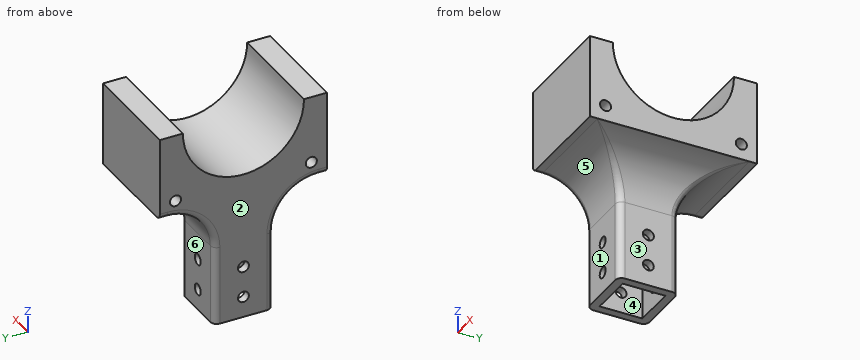
```python
from build123d import *

# Parameters (mm, degrees)
SKETCH_1_W          = 28.5
SKETCH_1_H          = 28.5
SKETCH_1_W_2        = 20.5
SKETCH_1_H_2        = 20.5
EXTRUDE_1_DEPTH     = 30
SKETCH_2_W          = 80
SKETCH_2_H          = 80
SKETCH_2_R          = 29
EXTRUDE_2_DEPTH     = 51
FILLET_1_R          = 22
CUT_EXTRUDE_1_DEPTH = 51
SKETCH_5_W          = 28.5
SKETCH_5_H          = 28.5
SKETCH_5_W_2        = 20.5
SKETCH_5_H_2        = 20.5
EXTRUDE_3_DEPTH     = 30
SKETCH_6_R          = 2.6
SKETCH_6_R_2        = 2.65
CUT_EXTRUDE_2_DEPTH = 30
SKETCH_7_R          = 2.65
CUT_EXTRUDE_3_DEPTH = 30
SKETCH_8_R          = 2.65
CUT_EXTRUDE_4_DEPTH = 96.399161422
FILLET_3_R          = 3


with BuildPart() as part:
    # 草图1 → 凸台-拉伸1 (new body)
    with BuildSketch(Plane.XY):
        Rectangle(SKETCH_1_W, SKETCH_1_H)
        Rectangle(SKETCH_1_W_2, SKETCH_1_H_2, mode=Mode.SUBTRACT)
    extrude(amount=EXTRUDE_1_DEPTH)

    # 草图2 → 凸台-拉伸2 (add)
    with BuildSketch(Plane.ZY.offset(14.25)):
        with Locations((70, 0)):
            Rectangle(SKETCH_2_W, SKETCH_2_H)
        with Locations((70, 0)):
            Circle(SKETCH_2_R, mode=Mode.SUBTRACT)
    extrude(amount=-EXTRUDE_2_DEPTH)

    # 圆角1
    fillet_1_edges = [part.edges().sort_by_distance(p)[0] for p in [
        (14.25, 0, 30),
        (0, 14.25, 30),
        (0, -14.25, 30),
    ]]
    fillet(fillet_1_edges, radius=FILLET_1_R)

    # 草图3 → 切除-拉伸1 (cut)
    with BuildSketch(Plane.ZY.offset(14.25)):
        with BuildLine():
            Line((70, -29), (70, -40))
            Line((70, -40), (110, -40))
            Line((110, -40), (110, 40))
            Line((110, 40), (70, 40))
            Line((70, 40), (70, 29))
            ThreePointArc((70, 29), (90.506096654, 20.506096654), (99, 0))
            ThreePointArc((99, 0), (90.506096654, -20.506096654), (70, -29))
        make_face()
    extrude(amount=-CUT_EXTRUDE_1_DEPTH, mode=Mode.SUBTRACT)

    # 草图5 → 凸台-拉伸3 (add)
    with BuildSketch(Plane(origin=(0, 0, 0), x_dir=(-1, 0, 0), z_dir=(0, 0, -1))):
        Rectangle(SKETCH_5_W, SKETCH_5_H)
        Rectangle(SKETCH_5_W_2, SKETCH_5_H_2, mode=Mode.SUBTRACT)
    extrude(amount=EXTRUDE_3_DEPTH)

    # 草图6 → 切除-拉伸2 (cut)
    with BuildSketch(Plane(origin=(14.25, 0, 0), x_dir=(0, 0, -1), z_dir=(1, 0, 0))):
        with Locations((20, 0)):
            Circle(SKETCH_6_R)
        with Locations((5, 0)):
            Circle(SKETCH_6_R_2)
    extrude(amount=-CUT_EXTRUDE_2_DEPTH, mode=Mode.SUBTRACT)

    # 草图7 → 切除-拉伸3 (cut)
    with BuildSketch(Plane(origin=(0, 14.25, 0), x_dir=(1, 0, 0), z_dir=(0, 1, 0))):
        with Locations(Location((0, 20, 0), (0, 0, 270))):
            Circle(SKETCH_7_R)
        with Locations(Location((0, 5, 0), (0, 0, 270))):
            Circle(SKETCH_7_R)
    extrude(amount=-CUT_EXTRUDE_3_DEPTH, mode=Mode.SUBTRACT)

    # 草图8 → 切除-拉伸4 (cut, through all)
    with BuildSketch(Plane.ZY.offset(14.25)):
        with Locations((37.5, 32.5)):
            Circle(SKETCH_8_R)
        with Locations((37.5, -32.5)):
            Circle(SKETCH_8_R)
    extrude(amount=-CUT_EXTRUDE_4_DEPTH, mode=Mode.SUBTRACT)

    # 圆角3
    fillet_3_edges = [part.edges().sort_by_distance(p)[0] for p in [
        (-14.25, -38.125, 30),
        (-14.25, 38.125, 30),
        (14.25, -14.25, -11),
        (-14.25, -14.25, -11),
        (14.25, 14.25, -11),
        (-14.25, 14.25, -11),
        (-14.25, -20.693650814, 23.556349186),
        (-14.25, 20.693650814, 23.556349186),
        (22.036924037, 22.036924037, 24.792512369),
        (22.036924037, -22.036924037, 24.792512369),
    ]]
    fillet(fillet_3_edges, radius=FILLET_3_R)


solid = part.part
```
Design review of the part built by this model. Coordinates are the model's own, in mm. Face numbers are marked on the shaded views. A direction names the side the tool comes from. Coordinates: 2 decimals unless noted, no trailing zeros. Order: outer loops, then holes, each group sorted by start corner. A loop starts at its lowest first (then second) coordinate and runs counter-clockwise, first axis right, second up. Notation, with made-up numbers: M 72.5,17.5 L 84.5,17.5 A31 cw 84.5,55.5 Z; hole C 58,59 d7. An arc over 180 degrees is marked long. Answer as a JSON object with one key per item and string values. Group by question number.
1) For pin 1 (4 mm diameter, centred on x = 0, z = -5, fed in from -Y); pin 2 (7 mm diameter, centred on x = 0, z = -20, fed in from -Y); pin 3 (6 mm diameter, centred on x = 3, z = 8.5, fed in from -Y); pin 4 (6 mm diameter, centred on y = -0.5, z = 10.5, fed in from +X), all flat-tipped, find the tip position at first contact; note any pin that passes through.
2) Add section A-A, the plane x = 0. Count the separate pieces of the cut face and the enclosed holes in it, then the cut area to 3 significant figures.
3) Mouldability with a two-part tool opening along X and no side actions: class the marked faces 1, 2, 3 and 4 as pulls with the +X half, pulls with the -X half, needs draft (parallel to the pull), parting line crosses it, or undercut.
4) Add section C-C, the plane z = -5. Write out the cut boundary in (x, y), then the cut area to 3 significant figures.
5) Add section B-B, the plane y = 0. Write out the cut boundary in (x, z).
6) Wall thickness on L1, parallel to Y at x = -0.5, z = -13; L2, parallel to Z at x = 4, y = 34.5; L3, parallel to Y at x = 12, z = -5: over which ranges is each line inside the solid? List them lowest first.
7) Add section D-D, the plane x = -8. Write out the cut boundary in (y, z), then the cut area to 3 significant figures.
8) Tool access review of the marked faces 5 and 6: name each direction out of +Z, -Z, +X, -X, +Y, -Y from which nothing blocks a thin tool from reaching the whole face with its end or side.
Computed values:
{
 "1": {"pin 1": "passes through", "pin 2": "stops at y = -14.25", "pin 3": "stops at y = -14.53", "pin 4": "stops at x = 14.95"},
 "2": {"separate pieces": "5", "enclosed holes": "2", "area": "2,440 mm^2"},
 "3": {"face 1": "needs draft", "face 2": "pulls with the -X half", "face 3": "pulls with the +X half", "face 4": "undercut"},
 "4": {"outline": "M -14.25,-11.25 A3 ccw -11.25,-14.25 L -2.65,-14.25 L -2.65,-10.25 L -10.25,-10.25 L -10.25,-2.65 L -14.25,-2.65 Z; M -14.25,2.65 L -10.25,2.65 L -10.25,10.25 L -2.65,10.25 L -2.65,14.25 L -11.25,14.25 A3 ccw -14.25,11.25 Z; M 2.65,-14.25 L 11.25,-14.25 A3 ccw 14.25,-11.25 L 14.25,-2.65 L 10.25,-2.65 L 10.25,-10.25 L 2.65,-10.25 Z; M 2.65,10.25 L 10.25,10.25 L 10.25,2.65 L 14.25,2.65 L 14.25,11.25 A3 ccw 11.25,14.25 L 2.65,14.25 Z", "area": "299 mm^2"},
 "5": {"outline": "M -14.25,-30 L -10.25,-30 L -10.25,-22.6 L -14.25,-22.6 Z; M -14.25,-17.4 L -10.25,-17.4 L -10.25,-7.65 L -14.25,-7.65 Z; M -14.25,-2.35 L -10.25,-2.35 L -10.25,30 L 10.25,30 L 10.25,-2.35 L 14.25,-2.35 L 14.25,8 A22 cw 36.25,30 L 36.75,30 L 36.75,41 L -14.25,41 Z; M 10.25,-30 L 14.25,-30 L 14.25,-22.6 L 10.25,-22.6 Z; M 10.25,-17.4 L 14.25,-17.4 L 14.25,-7.65 L 10.25,-7.65 Z"},
 "6": {"L1": "y = -14.25 to -10.25, 10.25 to 14.25", "L2": "z = 29.93 to 35.76, 39.24 to 70", "L3": "y = -14.15 to -2.65, 2.65 to 14.15"},
 "7": {"outline": "M -40,30 L -36.25,30 A22 cw -14.25,8 L -14.25,-30 L -10.25,-30 L -10.25,30 L 10.25,30 L 10.25,-30 L 14.25,-30 L 14.25,8 A22 cw 36.25,30 L 40,30 L 40,70 L 29,70 A29 cw -29,70 L -40,70 Z; hole C -32.5,37.5 d5.3; hole C 32.5,37.5 d5.3", "area": "2,520 mm^2"},
 "8": {"face 5": "-Z, +X, -X, -Y", "face 6": "-Z, +X, -X, +Y"}
}
